Input: dimensioned drawing with shaded views. Units: mm. Origin: part minimum x, y, z. A direction names the side the tool comes from. Give positions to 0.01 mm unless a question says otherwise; leave off trailing zeros. Loops run counter-clockwise (first coordinate to the right, second up) from the corner with the lowest first, then second, coordinate; pieces in that order, holes last. Notation, with made-up numbers: M 47.25,18 L 78.25,18 A25 cw 78.25,32 Z; hole C -31,62.25 d11. An arc over 180 degrees is marked long. Answer in a Markdown table with one row per item.
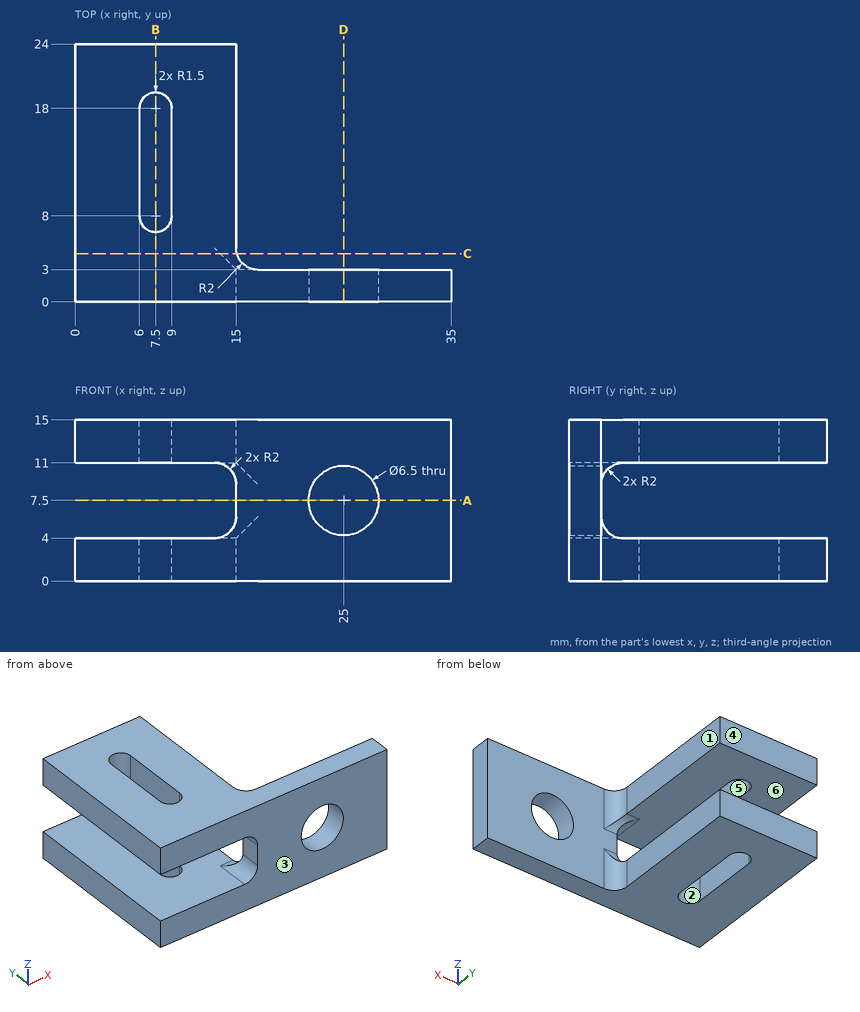
Q1. Mould query, pull axis Y, two halves, no side actions, for the marked faces 4, 5 and 6. Classes: +Y half, -Y half, draft (parallel to the pull), parting line (faces both ways), or undercut.
Values follow:
| item | result |
|---|---|
| face 4 | +Y half |
| face 5 | undercut |
| face 6 | draft |
Q2. Section query A-A (z = 7.5). Output: boundary loops of the cut face in (x, y), plus the area to 3 significant figures.
Values follow:
| item | result |
|---|---|
| outline | M 15,0 L 21.75,0 L 21.75,3 L 15,3 Z; M 28.25,0 L 35,0 L 35,3 L 28.25,3 Z |
| area | 40.5 mm^2 |
Q3. Reachability of the marked faces 1, 2 and 3 from +Z, -Z, +X, -X, +Y, -Y: full face, straight path, thin tool, end or side. Return the list, or none.
Values follow:
| item | result |
|---|---|
| face 1 | +Z, -Z, +X, +Y |
| face 2 | +Z, -Z |
| face 3 | +Z, -Z, +X, -X, -Y |
Q4. Contact query for flat-ended pins moving along their axis: pin 1 Ø1.2 at (y, z) = (10.5, 13.5) entering from +X; pin 2 Ø8 at (x, y) = (22.5, 21) entering from -Z; pin 3 Ø5 at (x, z) = (28, 11) entering from +Y; pin 4 Ø0.9 at (y, z) = (2, 7.5) entering from -X. Output: stop coordinate, or through.
Values follow:
| item | result |
|---|---|
| pin 1 | x = 15 |
| pin 2 | through |
| pin 3 | y = 3 |
| pin 4 | x = 15 |
Q5. Section query D-D (x = 25). Output: boundary loops of the cut face in (y, z).
Values follow:
| item | result |
|---|---|
| outline | M 0,0 L 3,0 L 3,4.25 L 0,4.25 Z; M 0,10.75 L 3,10.75 L 3,15 L 0,15 Z |
Q6. Section query C-C (y = 4.5). Output: boundary loops of the cut face in (x, z).
Values follow:
| item | result |
|---|---|
| outline | M 0,0 L 15.06,0 L 15.06,4.06 L 13.5,4.06 A2 cw 13,4 L 0,4 Z; M 0,11 L 13,11 A2 cw 13.5,10.94 L 15.06,10.94 L 15.06,15 L 0,15 Z |
Q7. Section query B-B (x = 7.5). Output: boundary loops of the cut face in (y, z), plus the area to 3 significant figures.
Values follow:
| item | result |
|---|---|
| outline | M 0,0 L 6.5,0 L 6.5,4 L 0,4 Z; M 0,11 L 6.5,11 L 6.5,15 L 0,15 Z; M 19.5,0 L 24,0 L 24,4 L 19.5,4 Z; M 19.5,11 L 24,11 L 24,15 L 19.5,15 Z |
| area | 88.0 mm^2 |
Q8. Ray query, probe 1 along X at (y, z) = (16, 1.5); probe 2 along Z at (x, y) = (25, 1.55); probe 3 along Z at (x, y) = (5, 21.5). Return the intervals inside material, ascending. Write a range as from..to.
Values follow:
| item | result |
|---|---|
| probe 1 | 0..6, 9..15 |
| probe 2 | 0..4.25, 10.75..15 |
| probe 3 | 0..4, 11..15 |
